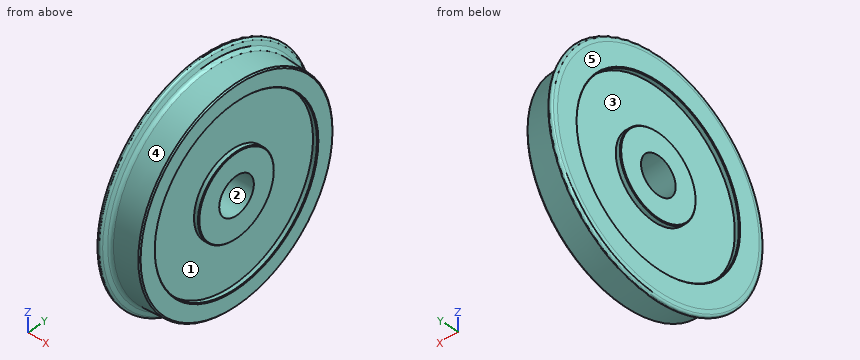
from build123d import *

# Parameters (mm, degrees)
F2_SIZE = 0.5
F4_D    = 16
F5_SIZE = 0.3


with BuildPart() as f1:
    # F0 (on Top) → F1 (revolve)
    with BuildSketch(Plane.XY):
        with BuildLine():
            Line((0, 17.5), (0, 0))
            Line((0, 0), (15, 0))
            Line((15, 0), (15, 17.5))
            Line((15, 17.5), (13, 17.5))
            Line((13, 17.5), (13, 37.5))
            Line((13, 37.5), (15, 37.5))
            Line((15, 37.5), (15, 44.83))
            Line((15, 44.83), (4.26, 45.35))
            ThreePointArc((4.26, 45.35), (3.3848643751, 45.7040621445), (2.84, 46.475))
            Line((2.84, 46.475), (2.26, 48.17))
            ThreePointArc((2.26, 48.17), (1.9775337426, 48.7058161582), (1.44, 48.985))
            ThreePointArc((1.44, 48.985), (0.6922694491, 48.8202067149), (0.28, 48.175))
            Line((0.28, 48.175), (0, 46.6))
            Line((0, 46.6), (0, 37.5))
            Line((0, 37.5), (2, 37.5))
            Line((2, 37.5), (2, 17.5))
            Line((2, 17.5), (0, 17.5))
        make_face()
    revolve(axis=Axis((7.5, 0, 0), (1, 0, 0)))

    # F2
    f2_edges = [f1.edges().sort_by_distance(p)[0] for p in [
        (15, -44.83, 0),
    ]]
    chamfer(f2_edges, length=F2_SIZE)

    # F4 (through all)
    with Locations(Plane(origin=(0, 0, 0), x_dir=(0, 1, 0), z_dir=(-1, 0, 0))):
        with Locations((0, 0)):
            Hole(F4_D / 2)

    # F5
    f5_edges = [f1.edges().sort_by_distance(p)[0] for p in [
        (15, -37.5, 0),
        (15, -17.5, 0),
        (0, -17.5, 0),
        (0, -37.5, 0),
    ]]
    chamfer(f5_edges, length=F5_SIZE)


solid = f1.part
The model under review builds one solid part; all positions refer to its coordinate system, in mm. Face numbers are marked on the shaded views. A direction names the side the tool comes from. Coordinates: 2 decimals unless noted, no trailing zeros. Loops run counter-clockwise (first coordinate to the right, second up) from the corner with the lowest first, then second, coordinate; pieces in that order, holes last.
(1) Wall thickness on L1, parallel to Z at x = 1.4, y = 0; L2, parallel to Z at x = 0.7, y = 0; L3, parallel to X at y = -36.5, z = 6: over which ranges is each line inside the solid? List them lowest first.
Determined:
L1: z = -48.99 to -37.5, -17.5 to -8, 8 to 17.5, 37.5 to 48.99
L2: z = -48.83 to -37.5, -17.5 to -8, 8 to 17.5, 37.5 to 48.83
L3: x = 2 to 13
(2) Insertion check: P1, Ø1.5, axis at x = 4, y = -21.5, coming from the -Z side; P2, Ø8, axis at y = 37, z = -38.5, coming from the +X side; P3, Ø2, axis at x = 7, y = -15.5, coming from the +Z side; P4, Ø1, axis at x = 1.5, y = 1, coming from the -Z side. Each pin has a flat end and moves straight along its axis. Give the tip position at first contact, or say it passes through.
Determined:
P1: stops at z = -40.56
P2: passes through
P3: stops at z = 42.83
P4: stops at z = -49
(3) Consider section A-A, the plane x = 5.75. Give the boundary of the cut face in (y, z).
Determined:
outline: circle Ø90.56 at (0, 0); hole circle Ø16 at (0, 0)
(4) Tool access review of the marked faces 1 and 2: name each direction out of +Z, -Z, +X, -X, +Y, -Y from which nothing blocks a thin tool from reaching the whole face with its end or side.
Determined:
face 1: +X
face 2: +X, -X
(5) Draft analysis for pull direction Z (two halves, no side actions). For the marked faces 3, 4 and 5, state which applies: +Z half, -Z half, draft (parallel to the pull), parting line (faces both ways), or undercut.
Determined:
face 3: undercut
face 4: parting line
face 5: draft
